The model under review builds one solid part; all positions refer to its coordinate system, in mm. Face numbers are marked on the shaded views. A direction names the side the tool comes from. Give positions to 0.01 mm unless a question says otherwise; leave off trailing zeros. Order: outer loops, then holes, each group sorted by start corner. A loop starts at its lowest first (then second) coordinate and runs counter-clockwise, first axis right, second up.
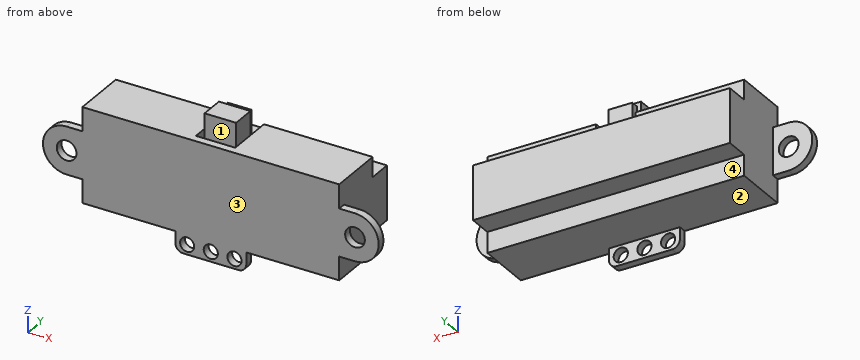
```python
from build123d import *

# Parameters (mm, degrees)
SKETCH1_W               = 32.576000126
SKETCH1_H               = 12
BOSS_EXTRUDE1_DEPTH     = 7
SKETCH2_W               = 32.576000126
SKETCH2_H               = 6.852850135
BOSS_EXTRUDE2_DEPTH     = 3
SKETCH3_R               = 0.9
BOSS_EXTRUDE3_DEPTH     = 1
BOSS_EXTRUDE5_START     = -1
BOSS_EXTRUDE5_OUTLINE_R = 1.25
BOSS_EXTRUDE5_DEPTH     = 1
SKETCH5_W               = 5
SKETCH5_H               = 2.525
CUT_EXTRUDE2_DEPTH      = 6
SKETCH6_W               = 4
SKETCH6_H               = 4
BOSS_EXTRUDE6_DEPTH     = 5
SKETCH7_W               = 4
SKETCH7_H               = 5
SKETCH7_W_2             = 3
SKETCH7_H_2             = 4
CUT_EXTRUDE4_DEPTH      = 1


# Read off the part's stored shape, not the designer's step: Boss-Extrude5
with BuildPart() as part:
    # Sketch1 → Boss-Extrude1 (new body)
    with BuildSketch(Plane(origin=(0, 0, 0), x_dir=(1, 0, 0), z_dir=(0, 1, 0))):
        with Locations((16.288000063, 6)):
            Rectangle(SKETCH1_W, SKETCH1_H)
    extrude(amount=BOSS_EXTRUDE1_DEPTH)

    # Sketch2 → Boss-Extrude2 (add)
    with BuildSketch(Plane(origin=(0, 7, 0), x_dir=(1, 0, 0), z_dir=(0, 1, 0))):
        with Locations((16.288000063, 5.951425068)):
            Rectangle(SKETCH2_W, SKETCH2_H)
    extrude(amount=BOSS_EXTRUDE2_DEPTH)

    # Sketch3 → Boss-Extrude3 (add)
    with BuildSketch(Plane.XZ):
        with BuildLine():
            ThreePointArc((19.788000063, -14.5), (20.495106844, -14.207106781), (20.788000063, -13.5))
            Line((20.788000063, -13.5), (20.788000063, -12))
            Line((20.788000063, -12), (11.788000063, -12))
            Line((11.788000063, -12), (11.788000063, -13.5))
            ThreePointArc((11.788000063, -13.5), (12.080893282, -14.207106781), (12.788000063, -14.5))
            Line((12.788000063, -14.5), (19.788000063, -14.5))
        make_face()
        with Locations(Location((13.288000063, -13.25, 0), (0, 0, 270))):
            Circle(SKETCH3_R, mode=Mode.SUBTRACT)
        with Locations(Location((16.288000063, -13.25, 0), (0, 0, 270))):
            Circle(SKETCH3_R, mode=Mode.SUBTRACT)
        with Locations(Location((19.288000063, -13.25, 0), (0, 0, 270))):
            Circle(SKETCH3_R, mode=Mode.SUBTRACT)
    extrude(amount=-BOSS_EXTRUDE3_DEPTH)

    # Boss-Extrude5 outline → Boss-Extrude5 (add)
    # profile 1 of 2: a face of its own
    with BuildSketch(Plane.XZ.offset(BOSS_EXTRUDE5_START)):
        with BuildLine():
            Line((32.576000126, -9.026382535), (34.576, -9.026382535))
            ThreePointArc((34.576, -9.026382535), (37.576, -6.026382535), (34.576, -3.026382535))
            Line((34.576, -3.026382535), (32.576000126, -3.026382535))
            Line((32.576000126, -3.026382535), (32.576000126, -9.026382535))
        make_face()
        with Locations((34.576, -6.026382535)):
            Circle(BOSS_EXTRUDE5_OUTLINE_R, mode=Mode.SUBTRACT)
    # profile 2 of 2: a face of its own
    with BuildSketch(Plane.XZ.offset(BOSS_EXTRUDE5_START)):
        with BuildLine():
            Line((-2, -9.026382535), (0, -9.026382535))
            Line((0, -9.026382535), (0, -3.026382535))
            Line((0, -3.026382535), (-2, -3.026382535))
            ThreePointArc((-2, -3.026382535), (-5, -6.026382535), (-2, -9.026382535))
        make_face()
        with Locations((-2, -6.026382535)):
            Circle(BOSS_EXTRUDE5_OUTLINE_R, mode=Mode.SUBTRACT)
    extrude(amount=BOSS_EXTRUDE5_DEPTH)

    # Sketch5 → Cut-Extrude2 (cut)
    with BuildSketch(Plane(origin=(0, 7, 0), x_dir=(1, 0, 0), z_dir=(0, 1, 0))):
        with Locations((16.288000063, 1.2625)):
            Rectangle(SKETCH5_W, SKETCH5_H)
    extrude(amount=-CUT_EXTRUDE2_DEPTH, mode=Mode.SUBTRACT)

    # Sketch6 → Boss-Extrude6 (add)
    with BuildSketch(Plane.XY.offset(-2.525)):
        with Locations((16.288000063, 4)):
            Rectangle(SKETCH6_W, SKETCH6_H)
    extrude(amount=BOSS_EXTRUDE6_DEPTH)

    # Sketch7 → Cut-Extrude4 (cut)
    with BuildSketch(Plane(origin=(0, 6, 0), x_dir=(1, 0, 0), z_dir=(0, 1, 0))):
        with Locations((16.288000063, 0.025)):
            Rectangle(SKETCH7_W, SKETCH7_H)
        with Locations((16.288000063, 0)):
            Rectangle(SKETCH7_W_2, SKETCH7_H_2, mode=Mode.SUBTRACT)
    extrude(amount=-CUT_EXTRUDE4_DEPTH, mode=Mode.SUBTRACT)


solid = part.part
```
1. Draft analysis for pull direction X (two halves, no side actions). For the marked faces 1 and 2, state which applies: pulls with the +X half, pulls with the -X half, needs draft (parallel to the pull), parting line crosses it, or undercut.
2. For the marked faces 3 and 4, list the 3-axis set-ups (+Z, -Z, +X, -X, +Y, -Y) from which the entire face can be reached by the end or side of a thin tool; tool diameter is ignored.
3. Take a section at D-D (x = 9.5). Write out the cut boundary in (y, z) (3 decimals).
4. Take a section at C-C (z = -13). Write out the cut boundary in (x, y).
5. Take a section at A-A (z = 0.5). Write out the cut boundary in (x, y).
6. Take a section at B-B (y = 4). Write out the cut boundary in (x, z) (3 decimals).
7. To check wall thickness, follow line 1 (X direction, y = 0.7, z = -13.25); line 2 (Y direction, x = 18, z = -2); line 3 (Z direction, x = 9, y = 3.5). State the ranges of each line that lie inside material, in increasing order.
8. Insertion check: pin 1 (5 mm diameter, centred on x = 13.5, y = 5.5, fed in from -Z); pin 2 (2.5 mm diameter, centred on x = -3, z = -6, fed in from +Y); pin 3 (1.5 mm diameter, centred on y = 3.5, z = -1, fed in from +X). Each pin has a flat end and moves straight along its axis. Give the tip position at first contact, or say it passes through.
Answer:
1. face 1: undercut
1. face 2: needs draft
2. face 3: +Z, -Z, +X, -X, -Y
2. face 4: -Z, +X, -X, +Y
3. outline: (0, -12) - (7, -12) - (7, -9.378) - (10, -9.378) - (10, -2.525) - (7, -2.525) - (7, 0) - (0, 0) - close
4. outline: (11.79, 0) - (12.42, 0) - (12.42, 1) - (11.79, 1) - close; (14.15, 0) - (15.42, 0) - (15.42, 1) - (14.15, 1) - close; (17.15, 0) - (18.42, 0) - (18.42, 1) - (17.15, 1) - close; (20.15, 0) - (20.79, 0) - (20.79, 1) - (20.15, 1) - close
5. outline: (14.29, 2) - (18.29, 2) - (18.29, 5) - (17.79, 5) - (17.79, 6) - (14.79, 6) - (14.79, 5) - (14.29, 5) - close
6. outline: (0, -12) - (32.576, -12) - (32.576, 0) - (18.788, 0) - (18.788, -2.525) - (18.288, -2.525) - (18.288, 2.475) - (14.288, 2.475) - (14.288, -2.525) - (13.788, -2.525) - (13.788, 0) - (0, 0) - close
7. line 1: x = 11.79 to 12.39, 14.19 to 15.39, 17.19 to 18.39, 20.19 to 20.79
7. line 2: y = 0 to 1, 2 to 5
7. line 3: z = -12 to 0
8. pin 1: stops at z = -12
8. pin 2: stops at y = 1
8. pin 3: stops at x = 32.58
